```python
from build123d import *

# Parameters (mm, degrees)
SKETCH_R     = 50
SKETCH_R_2   = 1.7
SKETCH_W     = 23
SKETCH_H     = 12
SKETCH_W_2   = 2
SKETCH_H_2   = 5.2
PAD_DEPTH    = 1
POCKET_DEPTH = 1.001


with BuildPart() as part:
    # Sketch → Pad (new body)
    with BuildSketch(Plane.XY):
        Circle(SKETCH_R)
        with Locations((-20.208313, -18.964277)):
            Circle(SKETCH_R_2, mode=Mode.SUBTRACT)
        with Locations((19.208313, -20.163197)):
            Circle(SKETCH_R_2, mode=Mode.SUBTRACT)
        with Locations((-23.214944, 31.641004)):
            Circle(SKETCH_R_2, mode=Mode.SUBTRACT)
        with Locations((25.194012, 33.188677)):
            Circle(SKETCH_R_2, mode=Mode.SUBTRACT)
        with Locations((0, -32)):
            Rectangle(SKETCH_W, SKETCH_H, mode=Mode.SUBTRACT)
        with Locations((21.708313, 1.054153)):
            Rectangle(SKETCH_W_2, SKETCH_H_2, mode=Mode.SUBTRACT)
        with Locations((21.708313, -8.945847)):
            Rectangle(SKETCH_W_2, SKETCH_H_2, mode=Mode.SUBTRACT)
        with Locations((-22.708313, -8.941766)):
            Rectangle(SKETCH_W_2, SKETCH_H_2, mode=Mode.SUBTRACT)
        with Locations((-22.708313, 1.058234)):
            Rectangle(SKETCH_W_2, SKETCH_H_2, mode=Mode.SUBTRACT)
    extrude(amount=PAD_DEPTH)

    # Sketch001 (on Face27 of Pad) → Pocket (cut, through all)
    with BuildSketch(Plane.XY.offset(1)):
        with BuildLine():
            Line((-42.708313, 26), (-42.708313, -26))
            ThreePointArc((-42.708313, 26), (-68.708313, 0), (-42.708313, -26))
        make_face()
        with BuildLine():
            Line((42.708313, 26), (42.708313, -26))
            ThreePointArc((42.708313, -26), (68.708313, 0), (42.708313, 26))
        make_face()
    extrude(amount=-POCKET_DEPTH, mode=Mode.SUBTRACT)


solid = part.part
```
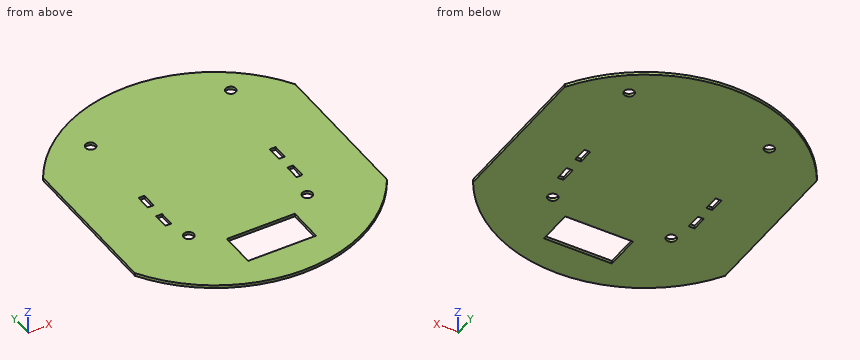
Read the model definition and answer for the solid it produces. Units are mm, in the model's axes. Coordinates: 2 decimals unless noted, no trailing zeros. Order: outer loops, then holes, each group sorted by start corner. A loop starts at its lowest first (then second) coordinate and runs counter-clockwise, first axis right, second up. Notation, with made-up numbers: (5.5, 61) - (12.5, 61) arc R13 cw to (12.5, 78) - close; hole circle Ø2 at (29, 74). An arc over 180 degrees is marked (long way). Answer as a JSON object with one key per item and string values. Group by question number.
Item 1: Consider probe 1 along X at (y, z) = (33, 0.15); probe 2 along X at (y, z) = (0, 0.5); probe 3 along Y at (x, z) = (-22, 0.1). Determine where each line is inside the solid, lowest interval first. Write a range as from..to.
Item 2: Section D-D (x = 33) is taken. Give the vertices of the cut face in (y, z), plus the area to 3 significant figures.
Item 3: Section A-A (y = 0) is taken. Give the vertices of the cut face in (x, z), plus the area to 3 significant figures.
Item 4: Section B-B (x = 5) is taken. Give the vertices of the cut face in (y, z).
Item 5: Flat-ended cylindrical pins translate along their axes: P1, Ø10, axis at x = 23, y = 39.5, coming from the -Z side; P2, Ø0.5, axis at x = -22.5, z = 0.5, coming from the -Y side; P3, Ø0.5, axis at x = -22.5, z = 0.5, coming from the +Y side; P4, Ø0.5, axis at x = 0.5, z = 0.5, coming from the -Y side. Find the tip coordinate at first contact, or state that the pin passes through.
Item 6: Section C-C (z = 0.7) is taken. State how many separate pieces and enclosed holes the cut face has, plus the area to 3 significant figures.
Results are:
{
 "1": {"probe 1": "x = -37.56..-24.24, -22.19..23.5, 26.88..37.56", "probe 2": "x = -42.71..-23.71, -21.71..20.71, 22.71..42.71", "probe 3": "y = -44.9..-11.54, -6.34..-1.54, 3.66..30.45, 32.83..44.9"},
 "2": {"outline": "(-37.56, 0) - (37.56, 0) - (37.56, 1) - (-37.56, 1) - close", "area": "75.1 mm^2"},
 "3": {"outline": "(-42.71, 0) - (-23.71, 0) - (-23.71, 1) - (-42.71, 1) - close; (-21.71, 0) - (20.71, 0) - (20.71, 1) - (-21.71, 1) - close; (22.71, 0) - (42.71, 0) - (42.71, 1) - (22.71, 1) - close", "area": "81.4 mm^2"},
 "4": {"outline": "(-49.75, 0) - (-38, 0) - (-38, 1) - (-49.75, 1) - close; (-26, 0) - (49.75, 0) - (49.75, 1) - (-26, 1) - close"},
 "5": {"P1": "stops at z = 0", "P2": "stops at y = -44.78", "P3": "stops at y = 44.78", "P4": "stops at y = -50"},
 "6": {"separate pieces": "1", "enclosed holes": "9", "area": "6,990 mm^2"}
}
